The model under review builds one solid part; all positions refer to its coordinate system, in mm. Round coordinates to 2 decimals unless told otherwise and drop trailing zeros. Order: outer loops, then holes, each group sorted by start corner. A loop starts at its lowest first (then second) coordinate and runs counter-clockwise, first axis right, second up.
from build123d import *

# Parameters (mm, degrees)
SKETCH1_W               = 25.4
SKETCH1_H               = 25.4
BOSS_EXTRUDE1_DEPTH     = 3.175
CUT_EXTRUDE1_DEPTH      = 19.238986403
CUT_EXTRUDE1_DEPTH_BACK = 19.238986403
SKETCH2_R               = 2.032


with BuildPart() as part:
    # Sketch1 → Boss-Extrude1 (new body)
    with BuildSketch(Plane.XY):
        Rectangle(SKETCH1_W, SKETCH1_H)
    extrude(amount=BOSS_EXTRUDE1_DEPTH)

    # Sketch2 → Cut-Extrude1 (cut, two sides: drawn at the far end of the back side and taken through both)
    with BuildSketch(Plane(origin=(0, 0, 0), x_dir=(-1, 0, 0), z_dir=(0, 0, -1)).offset(-CUT_EXTRUDE1_DEPTH_BACK)):
        with Locations((5.260512242, -7.756353865)):
            Circle(SKETCH2_R)
        with Locations((-6.35, -5.396866107)):
            Circle(SKETCH2_R)
        with Locations((-6.35, 7.303133893)):
            Circle(SKETCH2_R)
    extrude(amount=CUT_EXTRUDE1_DEPTH + CUT_EXTRUDE1_DEPTH_BACK, mode=Mode.SUBTRACT)


solid = part.part
(1) The part is to be moulded in two halves that separate along Y. For faces 1 (the flat face through (0, 12.7, 2)), 2 (the flat face through (0, -12.7, 2)), 3 (the cylindrical face through (-7.14, -8.53, 1.61)), 4 (the flat face through (12.7, 0, 2)), say which applies: pulls with the +Y half, pulls with the -Y half, needs draft (parallel to the pull), parting line crosses it, or undercut.
(2) We need section B-B (y = 8.25). Give the boundary of the cut face in (x, z) (3 decimals).
(3) We need section A-A (x = 6.35). Give the boundary of the cut face in (y, z) (3 decimals), and give its area (3 significant figures).
(4) To check wall thickness, follow L1, parallel to Y at x = 6.35, z = 1.6; L2, parallel to X at y = -6.5, z = 0.2; L3, parallel to X at y = -6.25, z = 1.05. State the ranges of each line that lie inside material, in increasing order.
(5) We need section D-D (y = -6.5). Give the boundary of the cut face in (x, z) (1 decimal), and give its area (3 significant figures).
(6) We need section C-C (x = -6). Give the boundary of the cut face in (y, z) (3 decimals).
Verdict:
1. face 1: pulls with the +Y half
1. face 2: pulls with the -Y half
1. face 3: undercut
1. face 4: needs draft
2. outline: (-12.7, 0) - (4.552, 0) - (4.552, 3.175) - (-12.7, 3.175) - close; (8.148, 0) - (12.7, 0) - (12.7, 3.175) - (8.148, 3.175) - close
3. outline: (-12.7, 0) - (-7.429, 0) - (-7.429, 3.175) - (-12.7, 3.175) - close; (-3.365, 0) - (5.271, 0) - (5.271, 3.175) - (-3.365, 3.175) - close; (9.335, 0) - (12.7, 0) - (12.7, 3.175) - (9.335, 3.175) - close
3. area: 54.8 mm2
4. L1: y = -12.7 to -7.43, -3.36 to 5.27, 9.34 to 12.7
4. L2: x = -12.7 to -6.86, -3.66 to 4.64, 8.06 to 12.7
4. L3: x = -12.7 to -6.62, -3.9 to 4.51, 8.19 to 12.7
5. outline: (-12.7, 0) - (-6.9, 0) - (-6.9, 3.2) - (-12.7, 3.2) - close; (-3.7, 0) - (4.6, 0) - (4.6, 3.2) - (-3.7, 3.2) - close; (8.1, 0) - (12.7, 0) - (12.7, 3.2) - (8.1, 3.2) - close
5. area: 59.7 mm2
6. outline: (-12.7, 0) - (-9.649, 0) - (-9.649, 3.175) - (-12.7, 3.175) - close; (-5.864, 0) - (12.7, 0) - (12.7, 3.175) - (-5.864, 3.175) - close
